Geometry: final body of the model. Coordinates: model frame, mm. A direction names the side the tool comes from. Round coordinates to 2 decimals unless told otherwise and drop trailing zeros. Loops run counter-clockwise (first coordinate to the right, second up) from the corner with the lowest first, then second, coordinate; pieces in that order, holes last. Notation, with made-up numbers: M -9.5,23 L 2.5,23 A13 ccw 2.5,40 Z; hole C 25,19.25 d3. An arc over 180 degrees is marked long. Write each question's results on one line, items separated by ' | '.
```python
from build123d import *

# Parameters (mm, degrees)
F1_DEPTH = 63.5
F2_DEPTH = 25.4
F3_DEPTH = 7.9375
F5_R     = 6.35


with BuildPart() as f1:
    # F0 (on Front) → F1 (new body, symmetric)
    with BuildSketch(Plane.XZ):
        Polygon((41.275, -9.525), (41.275, 9.525), (22.225, 9.525), (-41.275, 9.525), (-41.275, -9.525), align=None)
    extrude(amount=F1_DEPTH, both=True)

    # F0 (on Front) → F2 (join, symmetric)
    with BuildSketch(Plane.XZ):
        with BuildLine():
            Line((22.225, 9.525), (41.275, 9.525))
            Line((41.275, 9.525), (41.275, 27.0002))
            ThreePointArc((41.275, 27.0002), (45.92468, 38.22552), (57.15, 42.8752))
            Line((57.15, 42.8752), (60.325, 42.8752))
            Line((60.325, 42.8752), (60.325, 61.9252))
            Line((60.325, 61.9252), (57.15, 61.9252))
            add(Edge.make_bspline(
                [(57.15, 61.9252), (56.406917, 61.90542), (55.666126, 61.881815), (54.927698, 61.854425)],
                knots=[0, 0, 0, 0, 1.489577, 1.489577, 1.489577, 1.489577], degree=3))
            ThreePointArc((54.927698, 61.854425), (31.680709, 50.897289), (22.225, 27.0002))
            Line((22.225, 27.0002), (22.225, 9.525))
        make_face()
        Polygon((60.325, 61.9252), (60.325, 42.8752), (78.02037, 42.8752), (85.725, 42.8752), (85.725, 61.9252), (78.02037, 61.9252), align=None)
    extrude(amount=F2_DEPTH, both=True)

    # F0 (on Front) → F3 (join, symmetric)
    with BuildSketch(Plane.XZ):
        with BuildLine():
            Line((-41.275, 9.525), (22.225, 9.525))
            Line((22.225, 9.525), (22.225, 27.0002))
            ThreePointArc((22.225, 27.0002), (31.680709, 50.897289), (54.927698, 61.854425))
            add(Edge.make_bspline(
                [(54.927698, 61.854425), (0.389985, 59.831469), (-41.257529, 37.158326), (-41.275, 9.525)],
                knots=[1.489577, 1.489577, 1.489577, 1.489577, 111.504536, 111.504536, 111.504536, 111.504536], degree=3))
        make_face()
    extrude(amount=F3_DEPTH, both=True)

    # F0 (on Front) → F4 (revolve)
    with BuildSketch(Plane.XZ):
        Polygon((85.725, 42.8752), (85.725, 38.1), (111.125, 38.1), (111.125, 66.675), (85.725, 66.675), (85.725, 61.9252), align=None)
    revolve(axis=Axis((85.725, 0, 52.3875), (0, 0, 1)))

    # F5
    f5_edges = [f1.edges().sort_by_distance(p)[0] for p in [
        (41.275, -63.5, 0),
        (-41.275, -63.5, 0),
        (-41.275, 63.5, 0),
        (41.275, 63.5, 0),
    ]]
    fillet(f5_edges, radius=F5_R)


solid = f1.part
```
1. Access query for faces 1 (the face through (46, 25.4, 42)), 2 (the face through (46, -25.4, 42)), 3 (the face through (86, 0, 38.1)). Directions: +Z, -Z, +X, -X, +Y, -Y. A direction counts if a zero-diameter tool reaches every point of the face in a straight line with its end or side. Return the directions, or none.
Answer key:
face 1: +Z, +X, -X, +Y | face 2: +Z, +X, -X, -Y | face 3: -Z, +X, +Y, -Y
2. Draft query along X for faces 4 (the face through (60, 2, 42.875)), 5 (the face through (31.93, 16.55, 51.16)), 6 (the face through (0, 63.5, 0)). Return one class per face: pulls with the +X half, pulls with the -X half, needs draft (parallel to the pull), parting line crosses it, or undercut.
Answer key:
face 4: undercut | face 5: pulls with the -X half | face 6: needs draft
3. Section A-A (z = 4). Output: boundary loops of the cut face in (x, y) (3 decimals), then the cut area to 3 significant figures.
Answer key:
outline: M -41.275,-57.15 A6.35 ccw -34.925,-63.5 L 34.925,-63.5 A6.35 ccw 41.275,-57.15 L 41.275,57.15 A6.35 ccw 34.925,63.5 L -34.925,63.5 A6.35 ccw -41.275,57.15 Z | area: 10,400 mm²
4. Pin query (flat end, axial travel): P1, Ø1.5, axis at y = -3, z = 9, coming from the +X side (3 decimals); P2, Ø16.5, axis at x = -1, y = -39.5, coming from the +Z side (3 decimals); P3, Ø10, axis at y = 17, z = 41, coming from the -X side. Return the tip coordinate at first contact, or that it passes through.
Answer key:
P1: stops at x = 41.275 | P2: stops at z = 9.525 | P3: stops at x = 23.4
5. Section B-B (y = -28). Output: boundary loops of the cut face in (x, z) (3 decimals).
Answer key:
outline: M -41.275,-9.525 L 41.275,-9.525 L 41.275,9.525 L -41.275,9.525 Z
6. Ray query, probe 1 along X at (y, z) = (24, -4) (3 decimals); probe 2 along Y at (x, z) = (57, 48); probe 3 along Z at (x, y) = (16.5, 56) (3 decimals). Return the intervals inside material, ascending.
Answer key:
probe 1: x = -41.275 to 41.275 | probe 2: y = -25.4 to 25.4 | probe 3: z = -9.525 to 9.525
